CAD build for the part. Positions are in the model's coordinates, mm. A direction names the side the tool comes from. Give positions to 0.01 mm unless a question says otherwise; leave off trailing zeros. Write each loop counter-clockwise with the first axis right and the second up, starting at its lowest first coordinate (ties: lowest second). Pieces come first, ordered by that corner, then holes. Notation, with made-up numbers: (0, 21) - (24, 21) arc R20 cw to (24, 25) - close; hole circle Ø2 at (30, 71.25). An arc over 180 degrees is marked (long way). Answer as a JSON object with one key per item and string values.
from build123d import *

# Parameters (mm, degrees)
CROQUIS1_W              = 19
CROQUIS1_H              = 65
SALIENTE_EXTRUIR1_DEPTH = 23
CROQUIS2_R              = 3
SALIENTE_EXTRUIR2_DEPTH = 10
CROQUIS3_R              = 3
SALIENTE_EXTRUIR3_DEPTH = 39
CROQUIS4_R              = 1.5
SALIENTE_EXTRUIR4_DEPTH = 1


with BuildPart() as part:
    # Croquis1 → Saliente-Extruir1 (new body)
    with BuildSketch(Plane(origin=(0, 0, 0), x_dir=(1, 0, 0), z_dir=(0, 1, 0))):
        Rectangle(CROQUIS1_W, CROQUIS1_H)
    extrude(amount=SALIENTE_EXTRUIR1_DEPTH)

    # Croquis2 → Saliente-Extruir2 (add)
    with BuildSketch(Plane(origin=(9.5, 0, 0), x_dir=(0, 0, -1), z_dir=(1, 0, 0))):
        with Locations((21.5, 11.5)):
            Circle(CROQUIS2_R)
    extrude(amount=SALIENTE_EXTRUIR2_DEPTH)

    # Croquis3 → Saliente-Extruir3 (add)
    with BuildSketch(Plane(origin=(19.5, 0, 0), x_dir=(0, 0, -1), z_dir=(1, 0, 0))):
        with Locations((21.5, 11.5)):
            Circle(CROQUIS3_R)
    extrude(amount=-SALIENTE_EXTRUIR3_DEPTH)

    # Croquis4 → Saliente-Extruir4 (add)
    with BuildSketch(Plane.ZY.offset(9.5)):
        with Locations((-9.5, 11.962831391)):
            Circle(CROQUIS4_R)
    extrude(amount=SALIENTE_EXTRUIR4_DEPTH)


solid = part.part
Item 1: Cut at D-D (z = -9.5). Give the cut face in (x, y).
Entries:
{"outline": "(-10.5, 10.46) - (-9.5, 10.46) - (-9.5, 0) - (9.5, 0) - (9.5, 23) - (-9.5, 23) - (-9.5, 13.46) - (-10.5, 13.46) - close"}
Item 2: Which spindle directions (+Z, -Z, +X, -X, +Y, -Y) get a long thin tool onto all of the face, cutting with end or side? Do faces 5 (the cylindrical face through (-14.4, 11.6, -18.5)), 6 (the flat face through (-10.5, 12, -10)), 7 (the flat face through (0, 23, 0)). Say none if no direction does.
Entries:
{"face 5": "-X", "face 6": "+Z, -X, +Y, -Y", "face 7": "+Z, -Z, +X, -X, +Y"}
Item 3: Flat gauge pins, fed straight in: P1, Ø8, axis at y = 19, z = 11, coming from the +X side; P2, Ø0.9, axis at y = 12.5, z = -9, coming from the -X side; P3, Ø7, axis at y = 17, z = -4.5, coming from the -X side. Where does each tip first touch, or does it go through?
Entries:
{"P1": "x = 9.5", "P2": "x = -10.5", "P3": "x = -9.5"}
Item 4: Cut at C-C (y = 9.75). Give the cut face in (x, z).
Entries:
{"outline": "(-19.5, -23.94) - (-9.5, -23.94) - (-9.5, -32.5) - (9.5, -32.5) - (9.5, -23.94) - (19.5, -23.94) - (19.5, -19.06) - (9.5, -19.06) - (9.5, 32.5) - (-9.5, 32.5) - (-9.5, -19.06) - (-19.5, -19.06) - close"}
Item 5: Mould opens along Z. For faces 1 (the cylindrical face through (-9.993, 12.977, -10.606)), 2 (the flat face through (0, 11, 32.5)), 3 (the flat face through (0, 0, 0)), 4 (the cylindrical face through (14.4, 11.6, -18.5)) say: +Z half, -Z half, draft (parallel to the pull), parting line (faces both ways), or undercut.
Entries:
{"face 1": "undercut", "face 2": "+Z half", "face 3": "draft", "face 4": "parting line"}
Item 6: Probe line 1 (X direction, y = 3.5, z = -3); line 2 (Z direction, x = 10.5, y = 11.75); line 3 (Z direction, x = -13, y = 9). List the from-to ranges inside material, lowest first. Write a range as from..to.
Entries:
{"line 1": "-9.5..9.5", "line 2": "-24.49..-18.51", "line 3": "-23.16..-19.84"}
Item 7: Cut at A-A (z = -21.5). Give the cut face in (x, y).
Entries:
{"outline": "(-19.5, 8.5) - (-9.5, 8.5) - (-9.5, 0) - (9.5, 0) - (9.5, 8.5) - (19.5, 8.5) - (19.5, 14.5) - (9.5, 14.5) - (9.5, 23) - (-9.5, 23) - (-9.5, 14.5) - (-19.5, 14.5) - close"}
Item 8: Cut at B-B (x = 17). Give the cut face in (y, z), and give its area (3 significant figures).
Entries:
{"outline": "circle Ø6 at (11.5, -21.5)", "area": "28.3 mm2"}
